CAD build for the part. Positions are in the model's coordinates, mm. Give positions to 0.01 mm unless a question says otherwise; leave off trailing zeros. Loops run counter-clockwise (first coordinate to the right, second up) from the corner with the lowest first, then second, coordinate; pieces in that order, holes last.
Item 1: Saw through at B-B on z = 153. Give the cut face in (x, y).
Item 2: Probe probe 1 along Y at (x, z) = (12.25, 105.5); probe 2 along X at (y, z) = (16.25, 22). List the from-to ranges inside material, lowest first.
Item 3: Saw through at A-A on y = 16.75. Give the cut face in (x, z), plus the area to 3 significant figures.
Item 4: Saw through at C-C on z = 30. Give the cut face in (x, y).
Item 5: Drop a flat-ended pin along its axis: P1, Ø1.9, axis at x = 15, z = 221.45, coming from the +Y side. Give the stop position or say it passes through.
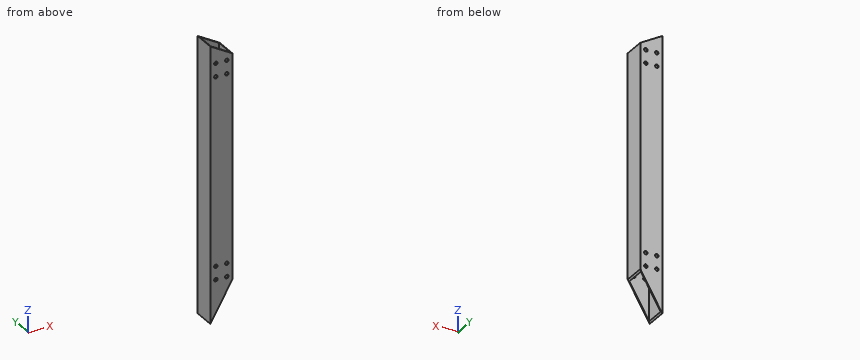
from build123d import *

# Parameters (mm, degrees)
SKETCH_1_W          = 20
SKETCH_1_H          = 20
SKETCH_1_W_2        = 18
SKETCH_1_H_2        = 18
EXTRUDE_1_DEPTH     = 250
CUT_EXTRUDE_1_DEPTH = 120
SKETCH_3_R          = 1.6
CUT_EXTRUDE_2_DEPTH = 252.594912508


with BuildPart() as part:
    # Sketch 1 → Extrude 1 (new body)
    with BuildSketch(Plane.XY):
        with Locations((10, 10)):
            Rectangle(SKETCH_1_W, SKETCH_1_H)
        with Locations((10, 10)):
            Rectangle(SKETCH_1_W_2, SKETCH_1_H_2, mode=Mode.SUBTRACT)
    extrude(amount=EXTRUDE_1_DEPTH)

    # Sketch 2 → Cut-Extrude 1 (cut)
    with BuildSketch(Plane(origin=(0, 20, 0), x_dir=(1, 0, 0), z_dir=(0, 1, 0))):
        Polygon((0, 0), (20, 0), (20, -34.641016151), align=None)
        Polygon((0, -250), (20, -238.452994616), (20, -250), align=None)
    extrude(amount=-CUT_EXTRUDE_1_DEPTH, mode=Mode.SUBTRACT)

    # Sketch 3 → Cut-Extrude 2 (cut, through all)
    with BuildSketch(Plane.XZ):
        with Locations(Location((5, 233.452994616, 0), (0, 0, 270))):
            Circle(SKETCH_3_R)
        with Locations(Location((15, 233.452994616, 0), (0, 0, 270))):
            Circle(SKETCH_3_R)
        with Locations(Location((15, 221.452994616, 0), (0, 0, 270))):
            Circle(SKETCH_3_R)
        with Locations(Location((5, 221.452994616, 0), (0, 0, 270))):
            Circle(SKETCH_3_R)
        with Locations(Location((15, 38.641016151, 0), (0, 0, 270))):
            Circle(SKETCH_3_R)
        with Locations(Location((5, 38.641016151, 0), (0, 0, 270))):
            Circle(SKETCH_3_R)
        with Locations(Location((15, 50.641016151, 0), (0, 0, 270))):
            Circle(SKETCH_3_R)
        with Locations(Location((5, 50.641016151, 0), (0, 0, 270))):
            Circle(SKETCH_3_R)
    extrude(amount=-CUT_EXTRUDE_2_DEPTH, mode=Mode.SUBTRACT)


solid = part.part
Results below:
1. outline: (0, 0) - (20, 0) - (20, 20) - (0, 20) - close; hole (1, 1) - (19, 1) - (19, 19) - (1, 19) - close
2. probe 1: y = 0 to 1, 19 to 20
2. probe 2: x = 0 to 1
3. outline: (0, 0) - (1, 1.73) - (1, 249.42) - (0, 250) - close; (19, 32.91) - (20, 34.64) - (20, 238.45) - (19, 239.03) - close
3. area: 454 mm2
4. outline: (0, 0) - (17.32, 0) - (17.32, 1) - (1, 1) - (1, 19) - (17.32, 19) - (17.32, 20) - (0, 20) - close
5. P1: passes through
